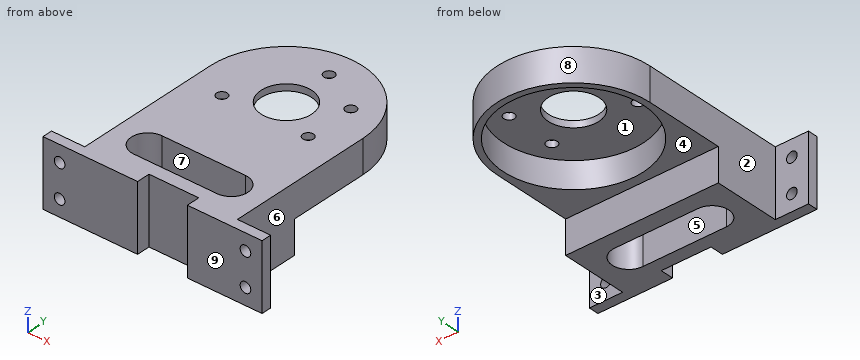
from build123d import *

# Parameters (mm, degrees)
EXTRUDE_1_DEPTH      = 20
CUT_EXTRUDE_1_DEPTH  = 10
SKETCH_3_R           = 21.1
CUT_EXTRUDE_2_DEPTH  = 8
SKETCH_7_R           = 1.6
CUT_EXTRUDE_6_DEPTH  = 3
SKETCH_8_R           = 7.6
CUT_EXTRUDE_7_DEPTH  = 3
SKETCH_12_W          = 46
SKETCH_12_H          = 20
EXTRUDE_4_DEPTH      = 20
SKETCH_14_W          = 10
SKETCH_14_H          = 20
SKETCH_14_R          = 1.6
EXTRUDE_5_DEPTH      = 3
SKETCH_16_W          = 15
SKETCH_16_H          = 20
CUT_EXTRUDE_10_DEPTH = 4
CUT_EXTRUDE_11_DEPTH = 61.811183182


with BuildPart() as part:
    # 草图1 → 凸台-拉伸1 (new body)
    with BuildSketch(Plane.XY):
        with BuildLine():
            Line((-23, 0), (-23, -27))
            Line((-23, -27), (23, -27))
            Line((23, -27), (23, 0))
            ThreePointArc((23, 0), (0, 23), (-23, 0))
        make_face()
    extrude(amount=EXTRUDE_1_DEPTH)

    # 草图2 → 切除-拉伸1 (cut)
    with BuildSketch(Plane(origin=(0, 0, 0), x_dir=(-1, 0, 0), z_dir=(0, 0, -1))):
        with BuildLine():
            Line((-23, -24), (23, -24))
            Line((23, -24), (23, 0))
            ThreePointArc((23, 0), (0, 23), (-23, 0))
            Line((-23, 0), (-23, -24))
        make_face()
    extrude(amount=-CUT_EXTRUDE_1_DEPTH, mode=Mode.SUBTRACT)

    # 草图3 → 切除-拉伸2 (cut)
    with BuildSketch(Plane(origin=(0, 0, 10), x_dir=(-1, 0, 0), z_dir=(0, 0, -1))):
        Circle(SKETCH_3_R)
    extrude(amount=-CUT_EXTRUDE_2_DEPTH, mode=Mode.SUBTRACT)

    # 草图7 → 切除-拉伸6 (cut)
    with BuildSketch(Plane.XY.offset(20)):
        with Locations((0, 15)):
            Circle(SKETCH_7_R)
        with Locations((12.990381057, 7.5)):
            Circle(SKETCH_7_R)
        with Locations((12.990381057, -7.5)):
            Circle(SKETCH_7_R)
        with Locations((-12.990381057, -7.5)):
            Circle(SKETCH_7_R)
    extrude(amount=-CUT_EXTRUDE_6_DEPTH, mode=Mode.SUBTRACT)

    # 草图8 → 切除-拉伸7 (cut)
    with BuildSketch(Plane(origin=(0, 0, 18), x_dir=(-1, 0, 0), z_dir=(0, 0, -1))):
        Circle(SKETCH_8_R)
    extrude(amount=-CUT_EXTRUDE_7_DEPTH, mode=Mode.SUBTRACT)

    # 草图12 → 凸台-拉伸4 (add)
    with BuildSketch(Plane.XZ.offset(27)):
        with Locations((0, 10)):
            Rectangle(SKETCH_12_W, SKETCH_12_H)
    extrude(amount=EXTRUDE_4_DEPTH)

    # 草图14 → 凸台-拉伸5 (add)
    # profile 1 of 2: a face of its own
    with BuildSketch(Plane.XZ.offset(47)):
        with Locations((28, 10)):
            Rectangle(SKETCH_14_W, SKETCH_14_H)
        with Locations(Location((28, 5, 0), (0, 0, 270))):
            Circle(SKETCH_14_R, mode=Mode.SUBTRACT)
        with Locations(Location((28, 15, 0), (0, 0, 270))):
            Circle(SKETCH_14_R, mode=Mode.SUBTRACT)
    # profile 2 of 2: a face of its own
    with BuildSketch(Plane.XZ.offset(47)):
        with Locations((-28, 10)):
            Rectangle(SKETCH_14_W, SKETCH_14_H)
        with Locations(Location((-28, 5, 0), (0, 0, 270))):
            Circle(SKETCH_14_R, mode=Mode.SUBTRACT)
        with Locations(Location((-28, 15, 0), (0, 0, 270))):
            Circle(SKETCH_14_R, mode=Mode.SUBTRACT)
    extrude(amount=-EXTRUDE_5_DEPTH)

    # 草图16 → 切除-拉伸10 (cut)
    with BuildSketch(Plane.XZ.offset(47)):
        with Locations((3, 10)):
            Rectangle(SKETCH_16_W, SKETCH_16_H)
    extrude(amount=-CUT_EXTRUDE_10_DEPTH, mode=Mode.SUBTRACT)

    # 草图17 → 切除-拉伸11 (cut, through all)
    with BuildSketch(Plane(origin=(0, 0, 0), x_dir=(-1, 0, 0), z_dir=(0, 0, -1))):
        with BuildLine():
            Line((-12.566151066, -29.028305096), (12.566151066, -29.028305096))
            ThreePointArc((12.566151066, -29.028305096), (17.53784597, -34), (12.566151066, -38.971694904))
            Line((12.566151066, -38.971694904), (-12.566151066, -38.971694904))
            ThreePointArc((-12.566151066, -38.971694904), (-17.53784597, -34), (-12.566151066, -29.028305096))
        make_face()
    extrude(amount=-CUT_EXTRUDE_11_DEPTH, mode=Mode.SUBTRACT)


solid = part.part
Check sheet for the modelled part. Datum: model origin and axes. Units: mm. Face numbers are marked on the shaded views. A direction names the side the tool comes from. Give positions to 0.01 mm unless a question says otherwise; leave off trailing zeros. Order: outer loops, then holes, each group sorted by start corner. A loop starts at its lowest first (then second) coordinate and runs counter-clockwise, first axis right, second up. Notation, with made-up numbers: M -28.75,70 L -3.75,70 A25 ccw -3.75,82 Z; hole C 56.25,53.5 d8. An arc over 180 degrees is marked long. Answer as CSV lines item,"result". Start each with the question number.
Item 1: Cross-section at D-D on x = -16. Enter the section's corners in (y, z), plus the area to 3 significant figures.
Item 2: Cross-section at C-C on z = 4.75. Enter the section's corners in (x, y).
Item 3: Tool access check on the marked faces 1, 2, 3, 4 and 5. Record the directions out of +Z, -Z, +X, -X, +Y, -Y that give a thin tool (end or side, any length) a straight path to the whole face; none if there is none.
Item 4: Cross-section at A-A on y = -34. Enter the section's corners in (x, z), plus the area to 3 significant figures.
Item 5: Cross-section at B-B on x = -28. Enter the section's corners in (y, z), plus the area to 3 significant figures.
Item 6: Gauge pin test, flat ends, axial feed: P1, Ø3, axis at x = 2, z = 13, coming from the -Y side; P2, Ø1.9, axis at x = -28, z = 5, coming from the -Y side; P3, Ø4, axis at y = -22.5, z = 8, coming from the -X side; P4, Ø12.5, axis at x = -10.5, y = 9.5, coming from the -Z side. Record the tip position at first contact, or that the pin passes through.
Item 7: Mould release check, pull along Y, two halves, no side actions. Record for the marked faces 6, 7, 8 and 9: +Y half, -Y half, draft (parallel to the pull), parting line (faces both ways), or undercut.
Item 8: Thickness scan on line 1 (X direction, y = -45.85, z = 15); line 2 (Y direction, x = 0, z = 18.5); line 3 (Y direction, x = -10, z = 2). Record the ranges inside material, lowest first. Write a range as [from, to].
Established:
1,outline,"M -47,0 L -37.6,0 L -37.6,20 L -47,20 Z; M -30.4,0 L -24,0 L -24,10 L -13.76,10 L -13.76,18 L 13.76,18 L 13.76,10 L 16.52,10 L 16.52,20 L -30.4,20 Z"
1,area,"501 mm^2"
2,outline,"M -33,-47 L -29.58,-47 L -29.58,-44 L -33,-44 Z; M -26.42,-47 L -4.5,-47 L -4.5,-43 L 10.5,-43 L 10.5,-47 L 26.42,-47 L 26.42,-44 L 23,-44 L 23,-24 L -23,-24 L -23,-44 L -26.42,-44 Z; M 29.58,-47 L 33,-47 L 33,-44 L 29.58,-44 Z; hole M -12.57,-38.97 L 12.57,-38.97 A4.97 ccw 12.57,-29.03 L -12.57,-29.03 A4.97 ccw Z"
3,face 1,"-Z"
3,face 2,"+Z, -Z, -X, +Y"
3,face 3,"+Z, -Z, +X, +Y"
3,face 4,"-Z, +X, -X, +Y"
3,face 5,"+Z, -Z"
4,outline,"M -23,0 L -17.54,0 L -17.54,20 L -23,20 Z; M 17.54,0 L 23,0 L 23,20 L 17.54,20 Z"
4,area,"218 mm^2"
5,outline,"M -47,0 L -44,0 L -44,3.4 L -47,3.4 Z; M -47,6.6 L -44,6.6 L -44,13.4 L -47,13.4 Z; M -47,16.6 L -44,16.6 L -44,20 L -47,20 Z"
5,area,"40.8 mm^2"
6,P1,"stops at y = -43"
6,P2,"passes through"
6,P3,"stops at x = -23"
6,P4,"stops at z = 18"
7,face 6,"draft"
7,face 7,"undercut"
7,face 8,"+Y half"
7,face 9,"-Y half"
8,line 1,"x = [-33, -29.6], [-26.4, -4.5], [10.5, 26.4], [29.6, 33]"
8,line 2,"y = [-43, -38.97], [-29.03, -7.6], [7.6, 13.4], [16.6, 23]"
8,line 3,"y = [-47, -38.97], [-29.03, -24]"
